from build123d import *

# Parameters (mm, degrees)
SHEET_EXTRUDE_DEPTH      = 31.8
M3_CLEARANCE_HOLE1_D     = 3.4
M3_CLEARANCE_HOLE1_DEPTH = 8.5
M3_CLEARANCE_HOLE1_TIP   = 1.021463052
M4_CLEARANCE_HOLE1_D     = 4.5
M4_CLEARANCE_HOLE1_DEPTH = 7.5
M4_CLEARANCE_HOLE1_TIP   = 1.351936393
FILLET1_R                = 10


with BuildPart() as part:
    # Sketch2 → Sheet Extrude (new body, symmetric)
    with BuildSketch(Plane(origin=(0, 0, 0), x_dir=(0, 0, -1), z_dir=(1, 0, 0))):
        Polygon((0, 0), (0, 2), (-35, 2), (-55, 2), (-115, 2), (-115, 0), (-55, 0), (-35, 0), align=None)
    extrude(amount=SHEET_EXTRUDE_DEPTH, both=True)

    # M3 Clearance Hole1
    with Locations(Plane(origin=(0, 2, 0), x_dir=(1, 0, 0), z_dir=(0, 1, 0))):
        with Locations((-24, -102.5), (-24, -86.5), (-8, -86.5), (-8, -102.5), (24, -102.5), (8, -102.5), (8, -86.5), (24, -86.5)):
            Hole(M3_CLEARANCE_HOLE1_D / 2, depth=M3_CLEARANCE_HOLE1_DEPTH)
            with Locations((0, 0, -(M3_CLEARANCE_HOLE1_DEPTH + M3_CLEARANCE_HOLE1_TIP / 2))):  # 118° drill point
                Cone(0, M3_CLEARANCE_HOLE1_D / 2, M3_CLEARANCE_HOLE1_TIP, mode=Mode.SUBTRACT)

    # M4 Clearance Hole1
    with Locations(Plane(origin=(0, 2, 0), x_dir=(1, 0, 0), z_dir=(0, 1, 0))):
        with Locations((0, -50.5), (22, -10.5), (-22, -10.5)):
            Hole(M4_CLEARANCE_HOLE1_D / 2, depth=M4_CLEARANCE_HOLE1_DEPTH)
            with Locations((0, 0, -(M4_CLEARANCE_HOLE1_DEPTH + M4_CLEARANCE_HOLE1_TIP / 2))):  # 118° drill point
                Cone(0, M4_CLEARANCE_HOLE1_D / 2, M4_CLEARANCE_HOLE1_TIP, mode=Mode.SUBTRACT)

    # Fillet1
    fillet1_edges = [part.edges().sort_by_distance(p)[0] for p in [
        (-31.8, 1, 0),
        (31.8, 1, 0),
    ]]
    fillet(fillet1_edges, radius=FILLET1_R)


solid = part.part
Design review of the part built by this model. Coordinates are the model's own, in mm. Coordinates: 2 decimals unless noted, no trailing zeros. Order: outer loops, then holes, each group sorted by start corner. A loop starts at its lowest first (then second) coordinate and runs counter-clockwise, first axis right, second up. Notation, with made-up numbers: (47.5, 7) -> (82.5, 7) arc R23 cw to (82.5, 32) -> close; hole circle Ø11 at (-22, 1.5). An arc over 180 degrees is marked (long way). Use one line per item in the form item = value. Start each with the question number.
(1) The part is to be moulded in two halves that separate along X. For faces 1 (the cylindrical face through (0.29, 0.99, 48.27)), 2 (the flat face through (31.8, 1, 63)), 3 (the flat face through (0, 1, 115)), say which applies: +X half, -X half, draft (parallel to the pull), parting line (faces both ways), or undercut.
(2) Add section B-B on x = 8. State the section outline as (y, z) points.
(3) For probe 1 along X at (y, z) = (0.45, 86.5); probe 2 along Z at (x, y) = (8, 1.1); probe 3 along X at (y, z) = (0.55, 10.5), list the stretches that pass through material, from the lowest coordinate up.
(4) Add section D-D on x = 0. State the section outline as (y, z) points.
(5) Insertion check: pin 1 (3 mm diameter, centred on x = -24, z = 102.5, fed in from +Y). The pin has a flat end and moves straight along its axis. Give the tip position at first contact, or say it passes through.
(6) Add section C-C on y = 0.95. Give the number of separate pieces and of enclosed holes in the cut face, plus the area to 3 significant figures.
(7) Add section A-A on z = 86.5. State the section outline as (x, y) points, plus the area to 3 significant figures.
Answer block:
q1.face_1 = undercut
q1.face_2 = +X half
q1.face_3 = draft
q2.outline = (0, 0) -> (2, 0) -> (2, 84.8) -> (0, 84.8) -> close; (0, 88.2) -> (2, 88.2) -> (2, 100.8) -> (0, 100.8) -> close; (0, 104.2) -> (2, 104.2) -> (2, 115) -> (0, 115) -> close
q3.probe_1 = -31.8 to -25.7, -22.3 to -9.7, -6.3 to 6.3, 9.7 to 22.3, 25.7 to 31.8
q3.probe_2 = 0 to 84.8, 88.2 to 100.8, 104.2 to 115
q3.probe_3 = -31.8 to -24.25, -19.75 to 19.75, 24.25 to 31.8
q4.outline = (0, 0) -> (2, 0) -> (2, 48.25) -> (0, 48.25) -> close; (0, 52.75) -> (2, 52.75) -> (2, 115) -> (0, 115) -> close
q5.pin_1 = through
q6.separate_pieces = 1
q6.enclosed_holes = 11
q6.area = 7,150 mm²
q7.outline = (-31.8, 0) -> (-25.7, 0) -> (-25.7, 2) -> (-31.8, 2) -> close; (-22.3, 0) -> (-9.7, 0) -> (-9.7, 2) -> (-22.3, 2) -> close; (-6.3, 0) -> (6.3, 0) -> (6.3, 2) -> (-6.3, 2) -> close; (9.7, 0) -> (22.3, 0) -> (22.3, 2) -> (9.7, 2) -> close; (25.7, 0) -> (31.8, 0) -> (31.8, 2) -> (25.7, 2) -> close
q7.area = 100 mm²
